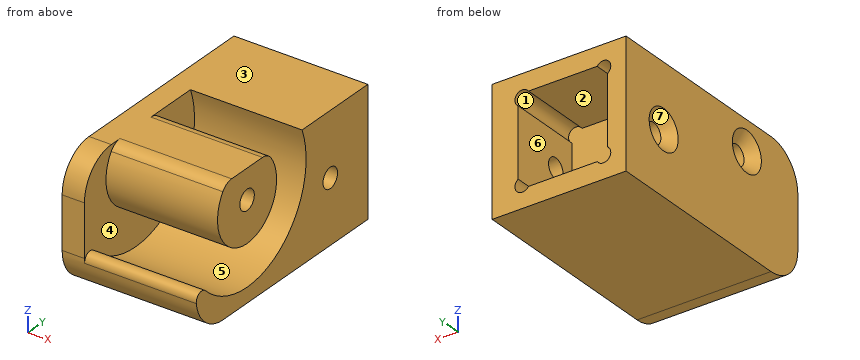
```python
from build123d import *

# Parameters (mm, degrees)
SKETCH_1_W                = 18
SKETCH_1_H                = 17
SKETCH_1_W_2              = 12
SKETCH_1_H_2              = 12
EXTRUDE_1_DEPTH           = 10
SKETCH_4_W                = 18
SKETCH_4_H                = 17
EXTRUDE_2_DEPTH           = 22
SKETCH_5_R                = 11
CUT_EXTRUDE_1_DEPTH       = 15
SKETCH_8_R                = 1.25
EXTRUDE_3_DEPTH           = 15
SKETCH_13_R               = 1.25
CUT_EXTRUDE_5_DEPTH       = 30.669007398
SKETCH_9_R                = 1.35
CUT_EXTRUDE_3_DEPTH       = 30.669007398
FILLET_4_R                = 5
SKETCH_20_R               = 1
CUT_EXTRUDE_7_DEPTH       = 10
FILLET_5_R                = 5
FILLET_6_R                = 2
FILLET_7_R                = 1
HOLE_WIZARD_1_D           = 2.7
HOLE_WIZARD_1_CSINK_D     = 5.4
HOLE_WIZARD_1_CSINK_ANGLE = 90


with BuildPart() as part:
    # 草图1 → 凸台-拉伸1 (new body)
    with BuildSketch(Plane(origin=(0, 0, 0), x_dir=(1, 0, 0), z_dir=(0, 1, 0))):
        Rectangle(SKETCH_1_W, SKETCH_1_H)
        with Locations((-0.5, 0)):
            Rectangle(SKETCH_1_W_2, SKETCH_1_H_2, mode=Mode.SUBTRACT)
    extrude(amount=EXTRUDE_1_DEPTH)

    # 草图4 → 凸台-拉伸2 (add)
    with BuildSketch(Plane.XZ):
        Rectangle(SKETCH_4_W, SKETCH_4_H)
    extrude(amount=EXTRUDE_2_DEPTH)

    # 草图5 → 切除-拉伸1 (cut)
    with BuildSketch(Plane.ZY.offset(-9)):
        with Locations((4.5, -12.5)):
            Circle(SKETCH_5_R)
    extrude(amount=CUT_EXTRUDE_1_DEPTH, mode=Mode.SUBTRACT)

    # 草图8 → 凸台-拉伸3 (add)
    with BuildSketch(Plane(origin=(-6, 0, 0), x_dir=(0, 0, -1), z_dir=(1, 0, 0))):
        with BuildLine():
            Line((-8.5, -8.725082782), (-8.5, -16.274917218))
            ThreePointArc((-8.5, -16.274917218), (1, -12.5), (-8.5, -8.725082782))
        make_face()
        with Locations(Location((-4.5, -12.5, 0), (0, 0, 180))):
            Circle(SKETCH_8_R, mode=Mode.SUBTRACT)
    extrude(amount=EXTRUDE_3_DEPTH)

    # 草图13 → 切除-拉伸5 (cut, through all)
    with BuildSketch(Plane(origin=(9, 0, 0), x_dir=(0, 0, -1), z_dir=(1, 0, 0))):
        with Locations((0, 3)):
            Circle(SKETCH_13_R)
    extrude(amount=-CUT_EXTRUDE_5_DEPTH, mode=Mode.SUBTRACT)

    # 草图9 → 切除-拉伸3 (cut, through all)
    with BuildSketch(Plane(origin=(9, 0, 0), x_dir=(0, 0, -1), z_dir=(1, 0, 0))):
        with Locations((-4.5, -12.5)):
            Circle(SKETCH_9_R)
    extrude(amount=-CUT_EXTRUDE_3_DEPTH, mode=Mode.SUBTRACT)

    # 圆角4
    fillet_4_edges = [part.edges().sort_by_distance(p)[0] for p in [
        (0, -22, -8.5),
    ]]
    fillet(fillet_4_edges, radius=FILLET_4_R)

    # 草图20 → 切除-拉伸7 (cut)
    with BuildSketch(Plane(origin=(0, 10, 0), x_dir=(1, 0, 0), z_dir=(0, 1, 0))):
        with Locations((4.944722215, -5.444722215)):
            Circle(SKETCH_20_R)
        with Locations((4.944722215, 5.444722215)):
            Circle(SKETCH_20_R)
        with Locations((-5.944722215, 5.444722215)):
            Circle(SKETCH_20_R)
        with Locations((-5.944722215, -5.444722215)):
            Circle(SKETCH_20_R)
    extrude(amount=-CUT_EXTRUDE_7_DEPTH, mode=Mode.SUBTRACT)

    # 圆角5
    fillet_5_edges = [part.edges().sort_by_distance(p)[0] for p in [
        (-7.5, -22, 8.5),
    ]]
    fillet(fillet_5_edges, radius=FILLET_5_R)

    # 圆角6
    fillet_6_edges = [part.edges().sort_by_distance(p)[0] for p in [
        (1.5, -16.274917218, 8.5),
        (1.5, -8.725082782, 8.5),
    ]]
    fillet(fillet_6_edges, radius=FILLET_6_R)

    # 圆角7
    # the kernel refuses this fillet: 1 mm, written as the material it takes off along each edge
    with BuildSketch(Plane(origin=(-6, -22, -1.045268253), x_dir=(0, 0.6114361728106764, -0.7912937549220469), z_dir=(1, 0, 0))) as fillet_7_piece_1:
        with BuildLine():
            CenterArc((2.970570235, -0.991624388), FILLET_7_R, 97.420778889, 142.097986779)
            Line((2.463314102, -1.853419733), (2.412588489, -1.939599267))
            ThreePointArc((2.412588489, -1.939599267), (1.881270284, -1.58004116), (-0.061143617, -0.079129375))
            Line((-0.061143617, -0.079129375), (0.012915523, 0.099162439))
            ThreePointArc((0.012915523, 0.099162439), (1.420707504, 0.00786827), (2.828499484, 0.099162439))
            Line((2.828499484, 0.099162439), (2.841415007, 0))
        make_face()
    extrude(amount=22.706766942, mode=Mode.SUBTRACT)

    # 打孔尺寸(%根据十字)槽沉头木螺钉的类型1 (through all)
    with Locations(Plane.ZY.offset(9)):
        with Locations((4.5, -12.5), (0, 3)):
            CounterSinkHole(HOLE_WIZARD_1_D / 2, HOLE_WIZARD_1_CSINK_D / 2, counter_sink_angle=HOLE_WIZARD_1_CSINK_ANGLE)


solid = part.part
```
The listing builds one solid part. Answer for the finished solid, in the listing's coordinates (mm). Face numbers are marked on the shaded views. A direction names the side the tool comes from. Coordinates: 2 decimals unless noted, no trailing zeros. Write each loop counter-clockwise with the first axis right and the second up, starting at its lowest first coordinate (ties: lowest second). Pieces come first, ordered by that corner, then holes. Notation, with made-up numbers: (-20, 79) - (31, 79) arc R23 cw to (31, 94) - close; hole circle Ø2 at (87, 45.25). An arc over 180 degrees is marked (long way). Return JSON: item names as keys, results as strings. Group by question number.
Q1. The part is cut by section D-D on z = 0. Write down the section's boundary in (x, y), and give its area (3 significant figures).
Q2. For a pull along X with two mould halves and no side action, classify the marked faces 1, 2, 3 and 4 as +X half, -X half, draft (parallel to the pull), parting line (faces both ways), or undercut.
Q3. The part is cut by section C-C on y = 8.5. Write down the section's boundary in (x, z), and give its area (3 significant figures).
Q4. Flat-ended cylindrical pins translate along their axes: pin 1 Ø1.8 at (x, z) = (4.94, 5.44) entering from +Y; pin 2 Ø1.5 at (y, z) = (4, -0.5) entering from -X; pin 3 Ø2.5 at (y, z) = (-12.5, 4.5) entering from -X; pin 4 Ø3.5 at (y, z) = (3, 0) entering from -X. Find the tip coordinate at first contact, or state that the pin passes through.
Q5. Which of the six approach directions +Z, -Z, +X, -X, +Y, -Y give full straight-line access (tool end or side, diameter ignored) to the marked faces 5, 6 and 7?
Q6. The part is cut by section A-A on y = -12.5. Write down the section's boundary in (x, z).
Q7. Find the intervals of material crossed by line 1 along X through (y, z) = (7, -0.5); line 2 along Y through (x, z) = (-6.95, 0); line 3 along Y through (x, z) = (7.75, 0), in increasing order. Write a range as [from, to].
Q8. The part is cut by section B-B on x = 3. Write down the section's boundary in (y, z).
Evaluation:
{
 "1": {"outline": "(-9, -22) - (-6, -22) - (-6, -15.66) - (9, -15.66) - (9, -9.34) - (-6, -9.34) - (-6, -2.46) - (9, -2.46) - (9, 1.65) - (5.5, 1.65) - (5.5, 0) - (-6.5, 0) - (-6.5, 1.65) - (-7.65, 1.65) - (-9, 0.3) - close; (-9, 5.7) - (-7.65, 4.35) - (-6.5, 4.35) - (-6.5, 10) - (-9, 10) - close; (5.5, 4.35) - (9, 4.35) - (9, 10) - (5.5, 10) - close", "area": "240 mm2"},
 "2": {"face 1": "undercut", "face 2": "undercut", "face 3": "draft", "face 4": "+X half"},
 "3": {"outline": "(-9, -8.5) - (9, -8.5) - (9, 8.5) - (-9, 8.5) - close; hole (-6.5, -4.61) arc R1 ccw (long way) to (-5.11, -6) - (4.11, -6) arc R1 ccw (long way) to (5.5, -4.61) - (5.5, 4.61) arc R1 ccw (long way) to (4.11, 6) - (-5.11, 6) arc R1 ccw (long way) to (-6.5, 4.61) - close", "area": "158 mm2"},
 "4": {"pin 1": "stops at y = 0", "pin 2": "stops at x = -8.17", "pin 3": "passes through", "pin 4": "stops at x = -8.05"},
 "5": {"face 5": "+X", "face 6": "+Y", "face 7": "-X"},
 "6": {"outline": "(-9, -8.5) - (9, -8.5) - (9, -6.5) - (-6, -6.5) - (-6, -1) - (9, -1) - (9, 3.15) - (-7.65, 3.15) - (-9, 1.8) - close; (-9, 7.2) - (-7.65, 5.85) - (9, 5.85) - (9, 8.5) - (-9, 8.5) - close"},
 "7": {"line 1": "x = [-9, -6.5], [5.5, 9]", "line 2": "y = [-22, 1.65], [4.35, 10]", "line 3": "y = [-15.66, -9.34], [-2.46, 1.65], [4.35, 10]"},
 "8": {"outline": "(-21.96, -4.13) arc R5 ccw to (-17, -8.5) - (10, -8.5) - (10, -6) - (0, -6) - (0, 6) - (10, 6) - (10, 8.5) - (-2.25, 8.5) arc R11 cw to (-20.26, -3.29) arc R1 ccw to start; (-17.01, 7.64) arc R5.5 ccw (long way) to (-7.99, 7.64) arc R2 ccw to (-9.63, 8.5) - (-15.37, 8.5) arc R2 ccw to start; hole circle Ø2.7 at (-12.5, 4.5)"}
}
